Work out the finished part from the listing and answer in its coordinate system (mm). A direction names the side the tool comes from. Round coordinates to 2 decimals unless told otherwise and drop trailing zeros. Write each loop counter-clockwise with the first axis right and the second up, starting at its lowest first coordinate (ties: lowest second). Pieces come first, ordered by that corner, then holes. Notation, with made-up numbers: M 61,-38.75 L 66,-38.75 A10 ccw 66,-20.75 Z; hole C 0,-29.5 d1. An arc over 180 degrees is marked long. One line per item, written item: value. Start each with the question number.
Q1. Consider probe 1 along Z at (x, y) = (30.5, 31); probe 2 along Y at (x, z) = (-13.5, 42.5); probe 3 along X at (y, z) = (-32.5, 44). Determine where each line is inside the solid, lowest interval first.
Q2. A tool of negligible diameter and unlimited length cuts with its end or side. For faces 4 (the flat face through (12.7, -13, 0)), 5 (the flat face through (-19, -12.7, 33)), 6 (the flat face through (0, -26, 38.1)), from which of +Z, -Z, +X, -X, +Y, -Y can it reach the whole face along a straight path? Write none if from no direction.
Q3. Given pin 1 Ø20.5 at (y, z) = (-23, 27) entering from +X; pin 2 Ø1.5 at (y, z) = (-8, 10.5) entering from -X; pin 3 Ø6 at (y, z) = (-18, 10.5) entering from +X, each flat-ended and moving along its own axis, determine where each tip first touches the part or whether it passes through.
Q4. Find section D-D (x = -21.5). Write down the section's boundary in (y, z).
Q5. Find section B-B (z = -8). Write down the section's boundary in (x, y), and give its area (3 significant figures).
Q6. The mould has two halves that part along Z. Classify faces 1 (the flat face through (1, 1, -12.7)), 2 (the flat face through (25, 12.7, 0)), 3 (the flat face through (-12.7, -26, 25)): released by +Z, released by -Z, zero draft, split by the parting line, or undercut.
Q7. Find section C-C (y = -17.5). Write down the section's boundary in (x, z).
Q8. Find section A-A (x = -9). Write down the section's boundary in (y, z).
from build123d import *

# Parameters (mm, degrees)
F0_W     = 25.4
F0_H     = 25.4
F1_DEPTH = 38.1
F2_W     = 25.4
F2_H     = 25.4
F3_DEPTH = 38.1
F4_W     = 25.4
F4_H     = 25.4
F5_DEPTH = 25.4
F6_W     = 25.4
F6_H     = 25.4
F7_DEPTH = 50.8
F8_W     = 25.4
F8_H     = 25.4
F9_DEPTH = 25.4


with BuildPart() as f1:
    # F0 (on Front) → F1 (new body, symmetric)
    with BuildSketch(Plane.XZ):
        Rectangle(F0_W, F0_H)
    extrude(amount=F1_DEPTH, both=True)

    # F2 (on Right) → F3 (join)
    with BuildSketch(Plane.YZ):
        with Locations((25.4, 0)):
            Rectangle(F2_W, F2_H)
    extrude(amount=F3_DEPTH)

    # F4 (on face) → F5 (join)
    with BuildSketch(Plane(origin=(-12.7, 0, 0), x_dir=(0, -1, 0), z_dir=(-1, 0, 0))):
        with Locations((25.4, 0)):
            Rectangle(F4_W, F4_H)
    extrude(amount=F5_DEPTH)

    # F6 (on face) → F7 (join)
    with BuildSketch(Plane.XY.offset(12.7)):
        with Locations((-25.4, -25.4)):
            Rectangle(F6_W, F6_H)
    extrude(amount=F7_DEPTH)

    # F8 (on face) → F9 (join)
    with BuildSketch(Plane.YZ.offset(-12.7)):
        with Locations((-25.4, 50.8)):
            Rectangle(F8_W, F8_H)
    extrude(amount=F9_DEPTH)


solid = f1.part
The answers:
1. probe 1: -12.7 to 12.7
1. probe 2: -38.1 to -12.7
1. probe 3: -38.1 to 12.7
2. face 4: +Z, -Z, +X, -Y
2. face 5: +Z, -X, +Y
2. face 6: +X, +Y, -Y
3. pin 1: x = -12.7
3. pin 2: x = -12.7
3. pin 3: x = 12.7
4. outline: M -38.1,-12.7 L -12.7,-12.7 L -12.7,63.5 L -38.1,63.5 Z
5. outline: M -38.1,-38.1 L 12.7,-38.1 L 12.7,12.7 L 38.1,12.7 L 38.1,38.1 L -12.7,38.1 L -12.7,-12.7 L -38.1,-12.7 Z
5. area: 3,230 mm2
6. face 1: released by -Z
6. face 2: zero draft
6. face 3: undercut
7. outline: M -38.1,-12.7 L 12.7,-12.7 L 12.7,12.7 L -12.7,12.7 L -12.7,38.1 L 12.7,38.1 L 12.7,63.5 L -38.1,63.5 Z
8. outline: M -38.1,-12.7 L 38.1,-12.7 L 38.1,12.7 L -38.1,12.7 Z; M -38.1,38.1 L -12.7,38.1 L -12.7,63.5 L -38.1,63.5 Z
